```python
from build123d import *

# Parameters (mm, degrees)
SKETCH_1_W             = 23.5
SKETCH_1_H             = 12
EXTRUDE_1_DEPTH        = 301
HOLE_WIZARD_M6_1_D     = 5
HOLE_WIZARD_M6_1_DEPTH = 15
HOLE_WIZARD_M6_1_TIP   = 1.502151548
HOLE_WIZARD_M6_2_D     = 5
HOLE_WIZARD_M6_2_DEPTH = 15
HOLE_WIZARD_M6_2_TIP   = 1.502151548
HOLE_WIZARD_M4_1_D     = 3.3
HOLE_WIZARD_M4_1_DEPTH = 10.1
HOLE_WIZARD_M4_1_TIP   = 0.991420021


with BuildPart() as part:
    # 草图1 → 凸台-拉伸1 (new, symmetric)
    with BuildSketch(Plane(origin=(0, 0, 0), x_dir=(0, 0, -1), z_dir=(1, 0, 0))):
        with BuildLine():
            Line((-14, 15), (-11.5, 15))
            Line((-11.5, 15), (-11.5, 13.5))
            Line((-11.5, 13.5), (-11.4, 13.5))
            ThreePointArc((-11.4, 13.5), (-11.117157288, 13.382842712), (-11, 13.1))
            Line((-11, 13.1), (-11, 12))
            Line((-11, 12), (-9.5, 12))
            Line((-9.5, 12), (-9.5, 15))
            Line((-9.5, 15), (-8, 15))
            Line((-8, 15), (-8, 12.5))
            Line((-8, 12.5), (-5, 12.5))
            Line((-5, 12.5), (-5, 15))
            Line((-5, 15), (5, 15))
            Line((5, 15), (5, 12.5))
            Line((5, 12.5), (8, 12.5))
            Line((8, 12.5), (8, 15))
            Line((8, 15), (9.5, 15))
            Line((9.5, 15), (9.5, 12))
            Line((9.5, 12), (11, 12))
            Line((11, 12), (11, 13.1))
            ThreePointArc((11, 13.1), (11.117157288, 13.382842712), (11.4, 13.5))
            Line((11.4, 13.5), (11.5, 13.5))
            Line((11.5, 13.5), (11.5, 15))
            Line((11.5, 15), (14, 15))
            ThreePointArc((14, 15), (14.707106781, 14.707106781), (15, 14))
            Line((15, 14), (15, 8))
            Line((15, 8), (12.5, 8))
            Line((12.5, 8), (12.5, 5))
            Line((12.5, 5), (15, 5))
            Line((15, 5), (15, -5))
            Line((15, -5), (12.5, -5))
            Line((12.5, -5), (12.5, -8))
            Line((12.5, -8), (15, -8))
            Line((15, -8), (15, -14))
            ThreePointArc((15, -14), (14.707106781, -14.707106781), (14, -15))
            Line((14, -15), (11.5, -15))
            Line((11.5, -15), (11.5, -13.5))
            Line((11.5, -13.5), (11.4, -13.5))
            ThreePointArc((11.4, -13.5), (11.117157288, -13.382842712), (11, -13.1))
            Line((11, -13.1), (11, -12))
            Line((11, -12), (9.5, -12))
            Line((9.5, -12), (9.5, -15))
            Line((9.5, -15), (8, -15))
            Line((8, -15), (8, -12.5))
            Line((8, -12.5), (5, -12.5))
            Line((5, -12.5), (5, -15))
            Line((5, -15), (-5, -15))
            Line((-5, -15), (-5, -12.5))
            Line((-5, -12.5), (-8, -12.5))
            Line((-8, -12.5), (-8, -15))
            Line((-8, -15), (-9.5, -15))
            Line((-9.5, -15), (-9.5, -12))
            Line((-9.5, -12), (-11, -12))
            Line((-11, -12), (-11, -13.1))
            ThreePointArc((-11, -13.1), (-11.117157288, -13.382842712), (-11.4, -13.5))
            Line((-11.4, -13.5), (-11.5, -13.5))
            Line((-11.5, -13.5), (-11.5, -15))
            Line((-11.5, -15), (-14, -15))
            ThreePointArc((-14, -15), (-14.707106781, -14.707106781), (-15, -14))
            Line((-15, -14), (-15, 14))
            ThreePointArc((-15, 14), (-14.707106781, 14.707106781), (-14, 15))
        make_face()
        with BuildLine():
            Line((12, -10.5), (12, -8.5))
            ThreePointArc((12, -8.5), (11.853553391, -8.146446609), (11.5, -8))
            Line((11.5, -8), (-11.5, -8))
            ThreePointArc((-11.5, -8), (-11.853553391, -8.146446609), (-12, -8.5))
            Line((-12, -8.5), (-12, -10.5))
            ThreePointArc((-12, -10.5), (-11.853553391, -10.853553391), (-11.5, -11))
            Line((-11.5, -11), (11.5, -11))
            ThreePointArc((11.5, -11), (11.853553391, -10.853553391), (12, -10.5))
        make_face(mode=Mode.SUBTRACT)
        with BuildLine():
            Line((-11.5, 11), (11.5, 11))
            ThreePointArc((11.5, 11), (11.853553391, 10.853553391), (12, 10.5))
            Line((12, 10.5), (12, 8.5))
            ThreePointArc((12, 8.5), (11.853553391, 8.146446609), (11.5, 8))
            Line((11.5, 8), (-11.5, 8))
            ThreePointArc((-11.5, 8), (-11.853553391, 8.146446609), (-12, 8.5))
            Line((-12, 8.5), (-12, 10.5))
            ThreePointArc((-12, 10.5), (-11.853553391, 10.853553391), (-11.5, 11))
        make_face(mode=Mode.SUBTRACT)
        Rectangle(SKETCH_1_W, SKETCH_1_H, mode=Mode.SUBTRACT)
    extrude(amount=EXTRUDE_1_DEPTH, both=True)

    # M6 螺纹孔1
    with Locations(Plane(origin=(0, 0, -15), x_dir=(-1, 0, 0), z_dir=(0, 0, -1))):
        with Locations((-281, 0), (-266, 0), (29, 0), (14, 0), (99, 0), (114, 0)):
            Hole(HOLE_WIZARD_M6_1_D / 2, depth=HOLE_WIZARD_M6_1_DEPTH)
            with Locations((0, 0, -(HOLE_WIZARD_M6_1_DEPTH + HOLE_WIZARD_M6_1_TIP / 2))):  # 118° drill point
                Cone(0, HOLE_WIZARD_M6_1_D / 2, HOLE_WIZARD_M6_1_TIP, mode=Mode.SUBTRACT)

    # M6 螺纹孔2
    with Locations(Plane(origin=(0, 15, 0), x_dir=(-1, 0, 0), z_dir=(0, 1, 0))):
        with Locations((281, 0), (266, 0), (-266, 0), (-281, 0)):
            Hole(HOLE_WIZARD_M6_2_D / 2, depth=HOLE_WIZARD_M6_2_DEPTH)
            with Locations((0, 0, -(HOLE_WIZARD_M6_2_DEPTH + HOLE_WIZARD_M6_2_TIP / 2))):  # 118° drill point
                Cone(0, HOLE_WIZARD_M6_2_D / 2, HOLE_WIZARD_M6_2_TIP, mode=Mode.SUBTRACT)

    # M4 螺纹孔1
    with Locations(Plane(origin=(0, 0, -15), x_dir=(-1, 0, 0), z_dir=(0, 0, -1))):
        with Locations((-96, 0), (-231, 0)):
            Hole(HOLE_WIZARD_M4_1_D / 2, depth=HOLE_WIZARD_M4_1_DEPTH)
            with Locations((0, 0, -(HOLE_WIZARD_M4_1_DEPTH + HOLE_WIZARD_M4_1_TIP / 2))):  # 118° drill point
                Cone(0, HOLE_WIZARD_M4_1_D / 2, HOLE_WIZARD_M4_1_TIP, mode=Mode.SUBTRACT)


solid = part.part
```
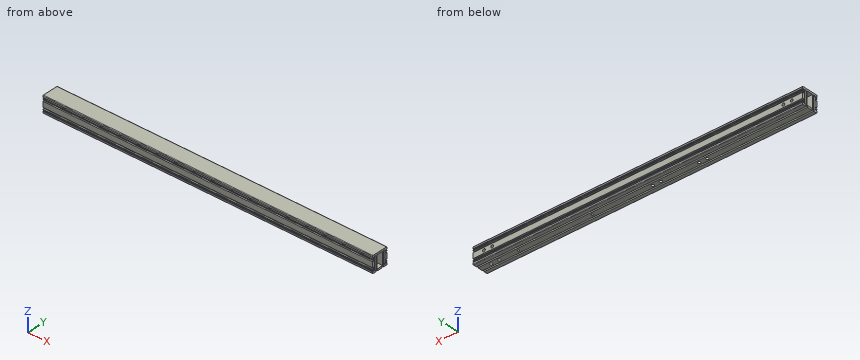
Input: part model. Units: mm. Frame: model coordinates. Round coordinates to 2 decimals unless told otherwise and drop trailing zeros. Answer as CSV lines item,"result".
1. Contact query for flat-ended pins moving along their axis: P1, Ø0.9, axis at x = 4, y = 6, coming from the -Z side; P2, Ø2.5, axis at x = -42.5, z = 6.5, coming from the -Y side. Output: stop coordinate, or through.
Geometry says:
P1,"stops at z = -12.5"
P2,"stops at y = -12.5"
2. Ray query, L1, parallel to Y at x = -29, z = -14.15; L2, parallel to Y at x = -177.5, z = -0.5; L3, parallel to Z at x = 266, y = 13.55. Return the intervals inside material, ascending. Write a range as [from, to].
Geometry says:
L1,"y = [-14.99, -8], [-5, -2.5], [2.5, 5], [8, 14.99]"
L2,"y = [-15, -11], [-8, -6], [6, 8], [11, 15]"
L3,"z = [-15, -11.5], [-9.5, -8], [-5, -2.5], [2.5, 5], [8, 9.5], [11.5, 15]"
3. Section A-A (x = 247). Give the number of separate pieces and of enclosed holes in the cut face, plus the area to 3 significant figures.
Geometry says:
separate pieces,"1"
enclosed holes,"3"
area,"407 mm^2"
